Input: part model. Units: mm. Frame: model coordinates. Face numbers are marked on the shaded views. A direction names the side the tool comes from. Round coordinates to 2 decimals unless told otherwise and drop trailing zeros. Order: outer loops, then holes, each group sorted by start corner. A loop starts at its lowest first (then second) coordinate and runs counter-clockwise, first axis right, second up. Notation, with made-up numbers: (-4, -32) -> (46, -32) arc R24 ccw to (46, -7) -> close; hole circle Ø9 at (-25, -14). An arc over 180 degrees is marked (long way). Answer as CSV lines item,"result". Start each with the question number.
1) Section query C-C, the plane z = 37. Output: boundary loops of the cut face in (x, y).
2) Section query A-A, the plane x = 0. Output: boundary loops of the cut face in (y, z).
3) Mould query, pull axis X, two halves, no side actions, for the marked faces 3, 4 and 5. Classes: +X half, -X half, draft (parallel to the pull), parting line (faces both ways), or undercut.
4) First-contact query: P1, Ø1.5, axis at x = 36, y = 35, coming from the +Z side; P2, Ø1, axis at x = -74, z = 22, coming from the -Y side; P3, Ø6, axis at x = 1.5, z = 27.5, coming from the -Y side. Flat tips, straight axial feed; report the tip coordinate or a pass-through.
5) Line query: L1, parallel to Y at x = 0.5, z = 4; L2, parallel to Y at x = 0, z = 13; L3, parallel to Z at x = -29.5, y = -52.5. Output: solid intervals per line, ascending.
6) Access query for the marked faces 1 and 2. Directions: +Z, -Z, +X, -X, +Y, -Y. A direction counts if a zero-diameter tool reaches every point of the face in a straight line with its end or side. Return the directions, or none.
7) Section query D-D, the plane y = 51.5. State how many separate pieces and enclosed holes the cut face has, and give its area (3 significant figures).
```python
from build123d import *

# Parameters (mm, degrees)
F0_R     = 37.69412
F1_DEPTH = 50.8
F0_R_2   = 95.718309
F2_DEPTH = 25.4
F3_R     = 8.619193
F4_DEPTH = 25.401
F5_R     = 21.217436
F6_DEPTH = 50.801
F7_R     = 5.08


with BuildPart() as f1:
    # F0 (on Top) → F1 (new body)
    with BuildSketch(Plane.XY):
        Circle(F0_R)
    extrude(amount=F1_DEPTH)

    # F0 (on Top) → F2 (join)
    with BuildSketch(Plane.XY):
        Circle(F0_R_2)
        Circle(F0_R, mode=Mode.SUBTRACT)
    extrude(amount=F2_DEPTH)

    # F3 (on face) → F4 (cut, through all)
    with BuildSketch(Plane.XY.offset(25.4)):
        with Locations((0, 76.732688)):
            Circle(F3_R)
        with Locations((-54.258204, 54.258204)):
            Circle(F3_R)
        with Locations((-76.732688, 0)):
            Circle(F3_R)
        with Locations((-54.258204, -54.258204)):
            Circle(F3_R)
        with Locations((0, -76.732688)):
            Circle(F3_R)
        with Locations((54.258204, -54.258204)):
            Circle(F3_R)
        with Locations((76.732688, 0)):
            Circle(F3_R)
        with Locations((54.258204, 54.258204)):
            Circle(F3_R)
    extrude(amount=-F4_DEPTH, mode=Mode.SUBTRACT)

    # F5 (on face) → F6 (cut, through all)
    with BuildSketch(Plane.XY.offset(50.8)):
        Circle(F5_R)
    extrude(amount=-F6_DEPTH, mode=Mode.SUBTRACT)

    # F7
    f7_edges = [f1.edges().sort_by_distance(p)[0] for p in [
        (-95.718309, 0, 25.4),
        (-37.69412, 0, 50.8),
        (-21.217436, 0, 50.8),
    ]]
    fillet(f7_edges, radius=F7_R)


solid = f1.part
```
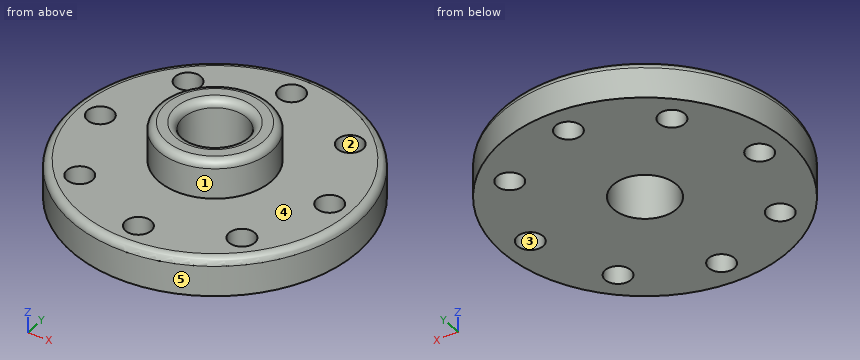
Findings:
1,outline,"circle Ø75.39 at (0, 0); hole circle Ø42.43 at (0, 0)"
2,outline,"(-95.72, 0) -> (-85.35, 0) -> (-85.35, 25.4) -> (-90.64, 25.4) arc R5.08 ccw to (-95.72, 20.32) -> close; (-68.11, 0) -> (-21.22, 0) -> (-21.22, 45.72) arc R5.08 ccw to (-26.3, 50.8) -> (-32.61, 50.8) arc R5.08 ccw to (-37.69, 45.72) -> (-37.69, 25.4) -> (-68.11, 25.4) -> close; (21.22, 0) -> (68.11, 0) -> (68.11, 25.4) -> (37.69, 25.4) -> (37.69, 45.72) arc R5.08 ccw to (32.61, 50.8) -> (26.3, 50.8) arc R5.08 ccw to (21.22, 45.72) -> close; (85.35, 0) -> (95.72, 0) -> (95.72, 20.32) arc R5.08 ccw to (90.64, 25.4) -> (85.35, 25.4) -> close"
3,face 3,"undercut"
3,face 4,"draft"
3,face 5,"parting line"
4,P1,"stops at z = 25.4"
4,P2,"stops at y = -60.92"
4,P3,"stops at y = -93.51"
5,L1,"y = -95.72 to -85.34, -68.13 to -21.21, 21.21 to 68.13, 85.34 to 95.72"
5,L2,"y = -95.72 to -85.35, -68.11 to -21.22, 21.22 to 68.11, 85.35 to 95.72"
5,L3,"z = 0 to 25.4"
6,face 1,"+Z"
6,face 2,"+Z, -Z"
7,separate pieces,"3"
7,enclosed holes,"0"
7,area,"3,260 mm^2"
